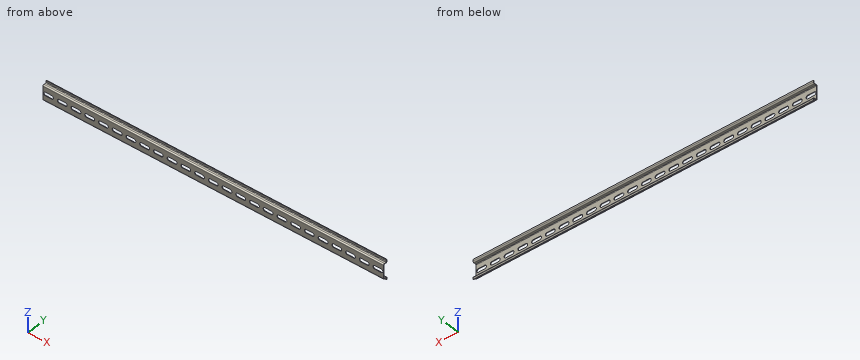
```python
from build123d import *

# Parameters (mm, degrees)
BASE_FLANGE1_DEPTH         = 310
EXTRUDE_CUT_DEPTH          = 311.561588095
LINEAR_PATTERN_1_COUNT     = 13
LINEAR_PATTERN_1_PITCH     = 25
LINEAR_PATTERN_1_COL_COUNT = 13
LINEAR_PATTERN_1_COL_PITCH = 25


# Sheet-metal steps are written as plain solids
with BuildPart() as part:
    # Sketch2 → Base-Flange1 (new, symmetric)
    with BuildSketch(Plane(origin=(0, 0, 0), x_dir=(0, 0, -1), z_dir=(1, 0, 0))):
        with BuildLine():
            Line((-17.5, 6.5), (-14.5, 6.5))
            ThreePointArc((-14.5, 6.5), (-13.792893219, 6.207106781), (-13.5, 5.5))
            Line((-13.5, 5.5), (-13.5, 2))
            ThreePointArc((-13.5, 2), (-12.914213562, 0.585786438), (-11.5, 0))
            Line((-11.5, 0), (11.5, 0))
            ThreePointArc((11.5, 0), (12.914213562, 0.585786438), (13.5, 2))
            Line((13.5, 2), (13.5, 5.5))
            ThreePointArc((13.5, 5.5), (13.792893219, 6.207106781), (14.5, 6.5))
            Line((14.5, 6.5), (17.5, 6.5))
            Line((17.5, 6.5), (17.5, 7.5))
            Line((17.5, 7.5), (14.5, 7.5))
            ThreePointArc((14.5, 7.5), (13.085786438, 6.914213562), (12.5, 5.5))
            Line((12.5, 5.5), (12.5, 2))
            ThreePointArc((12.5, 2), (12.207106781, 1.292893219), (11.5, 1))
            Line((11.5, 1), (-11.5, 1))
            ThreePointArc((-11.5, 1), (-12.207106781, 1.292893219), (-12.5, 2))
            Line((-12.5, 2), (-12.5, 5.5))
            ThreePointArc((-12.5, 5.5), (-13.085786438, 6.914213562), (-14.5, 7.5))
            Line((-14.5, 7.5), (-17.5, 7.5))
            Line((-17.5, 7.5), (-17.5, 6.5))
        make_face()
    extrude(amount=BASE_FLANGE1_DEPTH, both=True)

    # Sketch1 → Extrude Cut (cut, through all)
    with BuildSketch(Plane(origin=(0, 1, 0), x_dir=(1, 0, 0), z_dir=(0, 1, 0))):
        with BuildLine():
            Line((-5.85, 3.15), (5.85, 3.15))
            ThreePointArc((5.85, 3.15), (9, 0), (5.85, -3.15))
            Line((5.85, -3.15), (-5.85, -3.15))
            ThreePointArc((-5.85, -3.15), (-9, 0), (-5.85, 3.15))
        make_face()
    extrude_cut = extrude(amount=-EXTRUDE_CUT_DEPTH, mode=Mode.SUBTRACT)

    # Linear Pattern 1: Extrude Cut ×13
    with Locations(*[(i * LINEAR_PATTERN_1_PITCH, 0, 0) for i in range(1, LINEAR_PATTERN_1_COUNT)]):
        add(extrude_cut, mode=Mode.SUBTRACT)

    # Linear Pattern 1 col: Extrude Cut ×13
    with Locations(*[(-i * LINEAR_PATTERN_1_COL_PITCH, 0, 0) for i in range(1, LINEAR_PATTERN_1_COL_COUNT)]):
        add(extrude_cut, mode=Mode.SUBTRACT)


solid = part.part
```
The listing builds one solid part. Answer for the finished solid, in the listing's coordinates (mm). Give positions to 0.01 mm unless a question says otherwise; leave off trailing zeros. Order: outer loops, then holes, each group sorted by start corner. A loop starts at its lowest first (then second) coordinate and runs counter-clockwise, first axis right, second up. Notation, with made-up numbers: (11.25, 0.5) - (42.25, 0.5) arc R17 ccw to (42.25, 13.5) - close; hole circle Ø10 at (27.5, 68). An arc over 180 degrees is marked (long way). Answer in a Markdown table with one row per item. Add a question column.
Q1. Given P1, Ø1.1, axis at x = -172.5, y = 0.5, coming from the +Z side; P2, Ø1, axis at x = -134.5, y = 3, coming from the +Z side; P3, Ø0.5, axis at x = -152.5, y = 0.5, coming from the +Z side, each flat-ended and moving along its own axis, determine where each tip first touches the part or whether it passes through.
Q2. Find the intervals of material crossed by line 1 along Z through (x, y) = (207.5, 2); line 2 along Z through (x, y) = (-135, 7.25); line 3 along Y through (x, z) = (-14.5, 14.5), in increasing order. Write a range as [from, to].
Q3. The part is cut by section A-A (y = 4.25). Determine the outline of the cut face in (x, z), then the cut area to 3 significant figures.
Determined:
| question | item | result |
|---|---|---|
| 1 | P1 | stops at z = 13.26 |
| 1 | P2 | stops at z = 13.5 |
| 1 | P3 | stops at z = 13.06 |
| 2 | line 1 | z = [-13.5, -12.5], [12.5, 13.5] |
| 2 | line 2 | z = [-17.5, -13.53], [13.53, 17.5] |
| 2 | line 3 | y = [6.5, 7.5] |
| 3 | outline | (-310, -13.5) - (310, -13.5) - (310, -12.5) - (-310, -12.5) - close; (-310, 12.5) - (310, 12.5) - (310, 13.5) - (-310, 13.5) - close |
| 3 | area | 1,240 mm² |
